The listing builds one solid part. Answer for the finished solid, in the listing's coordinates (mm). Face numbers are marked on the shaded views. A direction names the side the tool comes from. Round coordinates to 2 decimals unless told otherwise and drop trailing zeros. Order: outer loops, then holes, each group sorted by start corner. A loop starts at its lowest first (then second) coordinate and runs counter-clockwise, first axis right, second up. Notation, with made-up numbers: (80, -35) -> (109, -35) arc R13 cw to (109, -18) -> close; hole circle Ø11 at (57, 20). An arc over 180 degrees is marked (long way). Answer in a Markdown table with one row per item. Add a question column.
```python
from build123d import *

# Parameters (mm, degrees)
SALIENTE_EXTRUIR2_DEPTH = 0.5
CORTAR_EXTRUIR1_DEPTH   = 0.5
CROQUIS10_R             = 1.5
SALIENTE_EXTRUIR5_DEPTH = 0.5
SALIENTE_EXTRUIR6_DEPTH = 6
SALIENTE_EXTRUIR8_DEPTH = 1


with BuildPart() as part:
    # Croquis2 → Saliente-Extruir2 (new body)
    with BuildSketch(Plane(origin=(0, 0, 0), x_dir=(1, 0, 0), z_dir=(0, 1, 0))):
        with BuildLine():
            Line((0, 0), (20, 0))
            Line((20, 0), (39.463577456, -4.600994744))
            ThreePointArc((39.463577456, -4.600994744), (39.040324802, 2.548287638), (34.753818463, 8.285642846))
            ThreePointArc((34.753818463, 8.285642846), (21.620038065, 13.895364206), (7.548005539, 11.457524625))
            ThreePointArc((7.548005539, 11.457524625), (2.056591074, 6.860161407), (0, 0))
        make_face()
    extrude(amount=SALIENTE_EXTRUIR2_DEPTH)

    # Croquis3 → Cortar-Extruir1 (cut)
    with BuildSketch(Plane(origin=(0, 0.5, 0), x_dir=(1, 0, 0), z_dir=(0, 1, 0))):
        with BuildLine():
            Line((20, 0), (16.5, 0))
            ThreePointArc((16.5, 0), (20.143291885, 1.229040833), (23.406126055, -0.80517408))
            Line((23.406126055, -0.80517408), (20, 0))
        make_face()
    extrude(amount=-CORTAR_EXTRUIR1_DEPTH, mode=Mode.SUBTRACT)

    # Croquis10 → Saliente-Extruir5 (add)
    with BuildSketch(Plane.XZ):
        Polygon((19.228440578, 6.617808668), (-0.235136993, 2.016814414), (0, 0), (19.62217394, -4.124844283), (39.463577456, 4.600994744), (39.228440578, 6.617808164), align=None)
        with Locations((19.622174052, 3.240683566)):
            Circle(CROQUIS10_R, mode=Mode.SUBTRACT)
    extrude(amount=-SALIENTE_EXTRUIR5_DEPTH)

    # Croquis11 → Saliente-Extruir6 (add)
    with BuildSketch(Plane(origin=(0, 0.5, 0), x_dir=(1, 0, 0), z_dir=(0, 1, 0))):
        Polygon((25.926575996, -3.088366571), (1.36009864, -1.814608984), (-0.235136987, -2.016814452), (19.228440593, -6.617808669), (39.228440593, -6.617808128), (40.823677784, -6.415602462), align=None)
    extrude(amount=SALIENTE_EXTRUIR6_DEPTH)

    # Croquis14 → Saliente-Extruir8 (add)
    with BuildSketch(Plane.XZ):
        with BuildLine():
            Line((39.463577456, 4.600994744), (39.228440578, 6.617808164))
            Line((39.228440578, 6.617808164), (19.228440578, 6.617808668))
            Line((19.228440578, 6.617808668), (-0.235136993, 2.016814414))
            Line((-0.235136993, 2.016814414), (0, 0))
            ThreePointArc((0, 0), (2.056591074, -6.860161407), (7.548005539, -11.457524625))
            ThreePointArc((7.548005539, -11.457524625), (21.620038065, -13.895364206), (34.753818463, -8.285642846))
            ThreePointArc((34.753818463, -8.285642846), (39.040324802, -2.548287638), (39.463577456, 4.600994744))
        make_face()
    extrude(amount=SALIENTE_EXTRUIR8_DEPTH)


solid = part.part
```
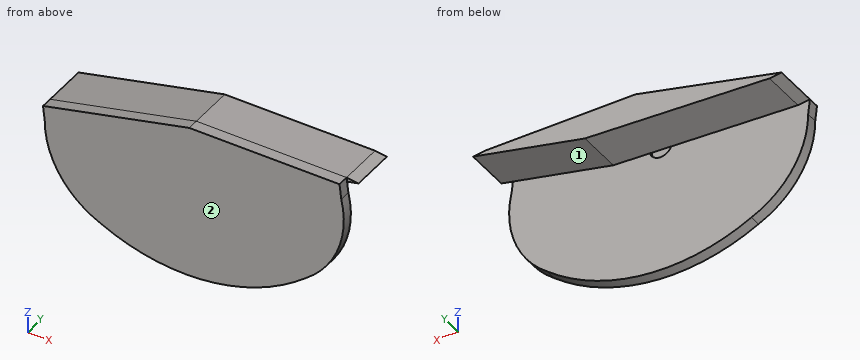
1. Straight lines are drawn through the part: line 1 along Y through (x, z) = (26, -2.5); line 2 along Z through (x, y) = (7.5, 5.75); line 3 along X through (y, z) = (-0.25, -2.5). For each, find the intervals that lie inside material, in ascending order.
2. The part is cut by section A-A (y = 1). Give the vertices of the cut face in (x, z).
3. Each of these flat-tipped pins is pushed along its axis until it touches: pin 1 (4 mm diameter, centred on x = 34, z = -10, fed in from +Y); pin 2 (1.5 mm diameter, centred on x = 25, y = 0.5, fed in from -Z). Where does it stop, or does it pass through?
4. The part is cut by section C-C (z = 5.25). Give the vertices of the cut face in (x, y), then the cut area to 3 significant figures.
5. The part is cut by section D-D (z = -11). Give the vertices of the cut face in (x, y).
6. The part is cut by section B-B (x = 8.5). Give the vertices of the cut face in (y, z).
7. For the marked faces 1 and 2, determine the directions among +Z, -Z, +X, -X, +Y, -Y from which every point of the face is accessible in a straight line to the end or side of a thin tool.
Report:
| question | item | result |
|---|---|---|
| 1 | line 1 | y = -1 to 0.5 |
| 1 | line 2 | z = 2.13 to 3.85 |
| 1 | line 3 | x = 0.25 to 39.06 |
| 2 | outline | (-0.24, 2.02) -> (1.36, 1.81) -> (25.93, 3.09) -> (40.82, 6.42) -> (39.23, 6.62) -> (19.23, 6.62) -> close |
| 3 | pin 1 | stops at y = 0.5 |
| 3 | pin 2 | stops at z = -13.45 |
| 4 | outline | (13.44, -1) -> (39.39, -1) -> (39.39, 0.5) -> (35.6, 0.5) -> (35.6, 6.5) -> (13.44, 6.5) -> close |
| 4 | area | 172 mm^2 |
| 5 | outline | (6.6, -1) -> (30.74, -1) -> (30.74, 0.5) -> (6.6, 0.5) -> close |
| 6 | outline | (-1, -11.9) -> (0.5, -11.9) -> (0.5, 2.18) -> (6.5, 2.18) -> (6.5, 4.08) -> (-1, 4.08) -> close |
| 7 | face 1 | -Z, +X, +Y |
| 7 | face 2 | +Z, -Z, +X, -X, -Y |
